Build history of the part. All positions in model axes, mm. A direction names the side the tool comes from. Round coordinates to 2 decimals unless told otherwise and drop trailing zeros. Write each loop counter-clockwise with the first axis right and the second up, starting at its lowest first coordinate (ties: lowest second). Pieces come first, ordered by that corner, then holes.
Item 1: Band-saw the part on A-A, the plane z = 143.5. Write the cut outline in (x, y), then the cut area to 3 significant figures.
Item 2: Band-saw the part on D-D, the plane z = 139. Write the cut outline in (x, y), then the cut area to 3 significant figures.
Item 3: Drop flat-ended pins along their axis: pin 1 Ø6 at (x, y) = (-5, 15) entering from -Z; pin 2 Ø1.8 at (x, z) = (-40, 134.5) entering from -Y; pin 3 Ø2.5 at (x, y) = (40, -6) entering from -Z. Give the stop position or say it passes through.
Item 4: Band-saw the part on B-B, the plane y = -25. Write the cut outline in (x, z).
Item 5: Wall check: probe 1 along X at (y, z) = (-25, 146.15); probe 2 along Y at (x, z) = (40, 145.6); probe 3 along X at (y, z) = (18.5, 143.5). Give the ranges that are in metal, low to high.
Item 6: 3-axis set-ups, long thin cutter, end or side, ignore diameter. For faces 1 (the flat face through (42, -5, 138)), 2 (the flat face through (-39, 7, 124.6)), 3 (the flat face through (41, 5, 130.5)): which of +Z, -Z, +X, -X, +Y, -Y reach the whole face in a straight line?
Item 7: Band-saw the part on C-C, the plane x = 40. Write the cut outline in (y, z), then the cut area to 3 significant figures.
Item 8: Mould opens along X. For faces 4 (the flat face through (41, -5, 130.5)), 5 (the flat face through (-1, -29.3, 144)) say: +X half, -X half, draft (parallel to the pull), parting line (faces both ways), or undercut.
```python
from build123d import *

# Parameters (mm, degrees)
SKETCH015_W             = 90
SKETCH015_H             = 60
SKETCH015_R             = 2
PAD009_DEPTH            = 2
SKETCH016_W             = 90.6
SKETCH016_H             = 60.6
SKETCH016_W_2           = 88.6
SKETCH016_H_2           = 58.6
PAD010_DEPTH            = 5
SKETCH017_W             = 6
SKETCH017_H             = 26.666667
PAD011_DEPTH            = 22.4
PAD014_START            = -3
PAD014_DEPTH            = 5
PAD015_START            = 3
PAD015_DEPTH            = 5
BODY004_PLACEMENT_ANGLE = 180


with BuildPart() as part:
    # Sketch015 → Pad009 (new body)
    with BuildSketch(Plane.XY):
        Rectangle(SKETCH015_W, SKETCH015_H)
        with Locations((-40, 25)):
            Circle(SKETCH015_R, mode=Mode.SUBTRACT)
        with Locations((-18, 25)):
            Circle(SKETCH015_R, mode=Mode.SUBTRACT)
        with Locations((40, 25)):
            Circle(SKETCH015_R, mode=Mode.SUBTRACT)
        with Locations((40, -25)):
            Circle(SKETCH015_R, mode=Mode.SUBTRACT)
        with Locations((-18, -25)):
            Circle(SKETCH015_R, mode=Mode.SUBTRACT)
        with Locations((-40, -25)):
            Circle(SKETCH015_R, mode=Mode.SUBTRACT)
    extrude(amount=PAD009_DEPTH)

    # Sketch016 → Pad010 (join)
    with BuildSketch(Plane.XY):
        Rectangle(SKETCH016_W, SKETCH016_H)
        Rectangle(SKETCH016_W_2, SKETCH016_H_2, mode=Mode.SUBTRACT)
    extrude(amount=PAD010_DEPTH)

    # Sketch017 → Pad011 (join)
    with BuildSketch(Plane.XY):
        with Locations((-38.7, -7.366666)):
            Rectangle(SKETCH017_W, SKETCH017_H)
    extrude(amount=PAD011_DEPTH)

    # Sketch020 → Pad014 (join)
    with BuildSketch(Plane.XZ.offset(PAD014_START)):
        Polygon((36, 0), (42, 0), (42, 16.5), (39, 16.5), (39, 5), align=None)
    extrude(amount=-PAD014_DEPTH)

    # Sketch020 → Pad015 (join)
    with BuildSketch(Plane.XZ.offset(PAD015_START)):
        Polygon((36, 0), (42, 0), (42, 16.5), (39, 16.5), (39, 5), align=None)
    extrude(amount=PAD015_DEPTH)


with BuildPart() as part_1:
    # Body004 placement: moved
    add(part.part.moved(Location((0, 0, 147))).rotate(Axis((0, 0, 147), (1, 0, 0)), BODY004_PLACEMENT_ANGLE))


solid = part_1.part
```
Results:
1. outline: (-45.3, -30.3) - (45.3, -30.3) - (45.3, 30.3) - (-45.3, 30.3) - close; (-41.7, -5.97) - (-35.7, -5.97) - (-35.7, 20.7) - (-41.7, 20.7) - close; (38.1, -8) - (42, -8) - (42, -3) - (38.1, -3) - close; (38.1, 3) - (42, 3) - (42, 8) - (38.1, 8) - close; hole (-44.3, -29.3) - (44.3, -29.3) - (44.3, 29.3) - (-44.3, 29.3) - close
1. area: 497 mm2
2. outline: (-41.7, -5.97) - (-35.7, -5.97) - (-35.7, 20.7) - (-41.7, 20.7) - close; (39, -8) - (42, -8) - (42, -3) - (39, -3) - close; (39, 3) - (42, 3) - (42, 8) - (39, 8) - close
2. area: 190 mm2
3. pin 1: stops at z = 145
3. pin 2: stops at y = -5.97
3. pin 3: stops at z = 130.5
4. outline: (-45.3, 142) - (-44.3, 142) - (-44.3, 145) - (-42, 145) - (-42, 147) - (-45.3, 147) - close; (-38, 145) - (-20, 145) - (-20, 147) - (-38, 147) - close; (-16, 145) - (38, 145) - (38, 147) - (-16, 147) - close; (42, 145) - (44.3, 145) - (44.3, 142) - (45.3, 142) - (45.3, 147) - (42, 147) - close
5. probe 1: x = -45.3 to -42, -38 to -20, -16 to 38, 42 to 45.3
5. probe 2: y = -30.3 to -27, -23 to 23, 27 to 30.3
5. probe 3: x = -45.3 to -44.3, -41.7 to -35.7, 44.3 to 45.3
6. face 1: -Z
6. face 2: -Z, +X, -X, +Y, -Y
6. face 3: -Z, +X, +Y, -Y
7. outline: (-30.3, 142) - (-29.3, 142) - (-29.3, 145) - (-27, 145) - (-27, 147) - (-30.3, 147) - close; (-23, 145) - (-8, 145) - (-8, 130.5) - (-3, 130.5) - (-3, 145) - (3, 145) - (3, 130.5) - (8, 130.5) - (8, 145) - (23, 145) - (23, 147) - (-23, 147) - close; (27, 145) - (29.3, 145) - (29.3, 142) - (30.3, 142) - (30.3, 147) - (27, 147) - close
7. area: 256 mm2
8. face 4: draft
8. face 5: undercut
